Read the model definition and answer for the solid it produces. Units are mm, in the model's axes. Coordinates: 2 decimals unless noted, no trailing zeros. Order: outer loops, then holes, each group sorted by start corner. A loop starts at its lowest first (then second) coordinate and runs counter-clockwise, first axis right, second up.
Solid Edge part; units mm, degrees
sketch "Sketch1" plane through (0, 0, 0) normal (1, 0, 0) x (0, 1, 0)
  line L0 (0, 180) -> (0, 0)
  line L1 (0, 0) -> (180, 0)
  line L2 (180, 0) -> (180, 20)
  line L3 (180, 20) -> (20, 20)
  line L4 (20, 20) -> (20, 180)
  line L5 (20, 180) -> (0, 180)
  dimension "D1" = 180
  dimension "D2" = 20
extrude "Protrusion1" add sketch "Sketch1" along normal mid plane 20
hole "hole_1" at (0, 20, 30) direction (0, -1, 0) diameter 3.75 end up to next start chamfer 0.6 start chamfer angle 45 end chamfer 0.6 end chamfer angle 45
pattern_linear "Pattern1" count 15 spacing 10 along (0, 0, 1) of "hole_1"
mirror "Mirror1" about plane through (0, 0, 0) normal (0, -0.7071, 0.7071) of "hole_1", "Pattern1"
properties material "Polyethylene (low density)"
1) A cutting plane is placed at A-A, the plane x = -7.25. Determine the outline of the cut face in (y, z).
A:
outline: (0, 0) - (180, 0) - (180, 20) - (20, 20) - (20, 180) - (0, 180) - close
2) Flat-ended cylindrical pins translate along their axes: pin 1 Ø4.5 at (x, z) = (0, 40) entering from +Y (3 decimals); pin 2 Ø3.5 at (x, z) = (0, 60) entering from +Y; pin 3 Ø5 at (x, y) = (0, 80) entering from +Z; pin 4 Ø4.5 at (x, y) = (0, 170) entering from +Z (3 decimals). Find the tip coordinate at first contact, or state that the pin passes through.
A:
pin 1: stops at y = 19.775
pin 2: passes through
pin 3: stops at z = 20
pin 4: stops at z = 19.775
3) A cutting plane is placed at B-B, the plane z = 135. Determine the outline of the cut face in (x, y).
A:
outline: (-10, 0) - (10, 0) - (10, 20) - (-10, 20) - close
4) Straight lines are drawn through the part: line 1 (X direction, y = 30, z = 14.25) (3 decimals); line 2 (Z direction, x = -5.5, y = 147.5). For each, find the intervals that lie inside material, in ascending order.
A:
line 1: x = -10 to -1.875, 1.875 to 10
line 2: z = 0 to 20
